The model under review builds one solid part; all positions refer to its coordinate system, in mm. A direction names the side the tool comes from. Round coordinates to 2 decimals unless told otherwise and drop trailing zeros. Order: outer loops, then holes, each group sorted by start corner. A loop starts at its lowest first (then second) coordinate and runs counter-clockwise, first axis right, second up. Notation, with made-up numbers: M 51,75 L 99,75 A18 ccw 99,106 Z; hole C 20.25,87 d11. An arc over 180 degrees is marked long. Use a Markdown table: item, result. Add a question column.
1. The part is to be moulded in two halves that separate along X. For faces 3 (the flat face through (-44.008, -8.908, 55.662)), 4 (the cylindrical face through (-14.31, -5.15, -55.94)), 5 (the flat face through (-44, -5, 56.914)), say which applies: +X half, -X half, draft (parallel to the pull), parting line (faces both ways), or undercut.
2. Insertion check: P1, Ø2, axis at y = -1.5, z = -33, coming from the -X side; P2, Ø2, axis at x = -40, z = -7, coming from the -Y side. Each pin has a flat end and moves straight along its axis. Give the tip position at first contact, or say it passes through.
3. For faces 1 (the flat face through (-45, -5, 54.374)), 2 (the cylindrical face through (-64.314, -1.252, 49.628)), list the 3-axis set-ups (+Z, -Z, +X, -X, +Y, -Y) from which the entire face can be reached by the end or side of a thin tool; tool diameter is ignored.
4. Consider section A-A on y = -6.5. State the section outline as (x, z) points.
5. To check wall thickness, follow probe 1 along Z at (x, y) = (-30, -3.25); probe 2 along X at (y, z) = (-3, 50); probe 3 along X at (y, z) = (-6.5, -52.5). State the ranges of each line that lie inside material, in increasing order.
6. Consider section B-B on x = -43. State the section outline as (y, z) points.
7. Consider section C-C on z = 15.5. State the section outline as (x, y) points.
from build123d import *

# Parameters (mm, degrees)
F1_DEPTH     = 12.7
F2_T         = -2.54
F3_R         = 5.08
F4_T1_DEPTH  = 109.2192415341
F4_T6_DEPTH  = 70.8878458195
F4_T11_DEPTH = 71.2857341695
F4_T16_DEPTH = 135.3482654479
F4_T23_DEPTH = 70.8878458195
F4_S24_R     = 5.08
F4_T25_DEPTH = 37
F4_T29_DEPTH = 135.3482654479
F4_S30_R     = 5.08
F4_T31_DEPTH = 69
F4_T38_DEPTH = 122.283391113
F4_S39_R     = 5.08
F4_T40_DEPTH = 63
F4_T44_DEPTH = 83.9519953984
F4_S45_R     = 5.08
F4_T46_DEPTH = 44
F4_T53_DEPTH = 84.3498837483
F4_S54_R     = 5.08
F4_T55_DEPTH = 44
F4_T59_DEPTH = 122.283391113
F4_S60_R     = 5.08
F4_T61_DEPTH = 63
F4_T68_DEPTH = 71.2857341695
F4_S69_R     = 5.08
F4_T70_DEPTH = 37
F4_T74_DEPTH = 135.3482654479
F4_S75_R     = 5.08
F4_T76_DEPTH = 69
F5_R         = 3.1205414485
F6_DEPTH     = 25.4


# Not quite as in the source:
# - a fillet or chamfer that OpenCascade refuses, or shapes differently, is made with other operations: its cross-section is extruded or revolved along the edge and cut away or added


with BuildPart() as f1:
    # F0 (on Front) → F1 (new body)
    with BuildSketch(Plane.XZ):
        Polygon((-76.0919898748, 56.9143295288), (-75.6755949615, -57.3849120053), (-12.7811351476, -57.3849120053), (-12.7811351476, 56.9143295288), align=None)
    extrude(amount=F1_DEPTH)

    # F2
    f2_openings = [f1.faces().sort_by_distance(p)[0] for p in [
        (-44.332578, -12.7, -0.172439),
    ]]
    offset(amount=F2_T, openings=f2_openings)

    # F3
    f3_edges = [f1.edges().sort_by_distance(p)[0] for p in [
        (-12.781135, -6.35, 56.91433),
        (-76.09199, -6.35, 56.91433),
        (-12.781135, -6.35, -57.384912),
        (-75.675595, -6.35, -57.384912),
    ]]
    fillet(f3_edges, radius=F3_R)

    # F4: chamfer of 5.08 on 4 edges, made by hand

    # F4_s2 → F4_t1 (cut)
    with BuildSketch(Plane.XY.offset(-54.8449120053)):
        Polygon((-10.2411351476, -12.7), (-15.3211351476, -7.62), (-15.3211351476, -12.7), align=None)
    extrude(amount=F4_T1_DEPTH, mode=Mode.SUBTRACT)


with BuildPart() as f4_tool4:
    # F4_s5 → F4_t6 (new body)
    with BuildSketch(Plane.YZ.offset(-86.2089809671)):
        Polygon((-12.7, -59.9249120053), (-7.62, -54.8449120053), (-12.7, -54.8449120053), align=None)
    extrude(amount=F4_T6_DEPTH)

    split(bisect_by=Plane(origin=(-73.3436593453, 0, -0.2671927326), x_dir=(0, 1, 0), z_dir=(0.9999933643, 0, 0.0036430001)), keep=Keep.TOP)


with BuildPart() as f1_1:
    add(f1.part)

    # F4_t3: cut F4_tool4
    add(f4_tool4.part, mode=Mode.SUBTRACT)


with BuildPart() as f4_tool9:
    # F4_s10 → F4_t11 (new body)
    with BuildSketch(Plane.YZ.offset(-15.3211351476)):
        Polygon((-12.7, 59.4543295288), (-7.62, 54.3743295288), (-12.7, 54.3743295288), align=None)
    extrude(amount=-F4_T11_DEPTH)

    split(bisect_by=Plane(origin=(-73.3436593453, 0, -0.2671927326), x_dir=(0, 1, 0), z_dir=(0.9999933643, 0, 0.0036430001)), keep=Keep.TOP)


with BuildPart() as f1_2:
    add(f1_1.part)

    # F4_t8: cut F4_tool9
    add(f4_tool9.part, mode=Mode.SUBTRACT)


with BuildPart() as f4_tool14:
    # F4_s15 → F4_t16 (new body)
    with BuildSketch(Plane(origin=(-0.2466530914, 0, 67.7055851499), x_dir=(0, 1, 0), z_dir=(0.0036430001, 0, -0.9999933643))):
        Polygon((-12.7, -78.4241460385), (-7.62, -73.3441460385), (-12.7, -73.3441460385), align=None)
    extrude(amount=F4_T16_DEPTH)

    split(bisect_by=Plane.XY.offset(54.3743295288), keep=Keep.BOTTOM)

    split(bisect_by=Plane.XY.offset(-54.8449120053), keep=Keep.TOP)


with BuildPart() as f1_3:
    add(f1_2.part)

    # F4_t13: cut F4_tool14
    add(f4_tool14.part, mode=Mode.SUBTRACT)


with BuildPart() as f4_tool21:
    # F4_s22 → F4_t23 (new body)
    with BuildSketch(Plane.YZ.offset(-86.2089809671)):
        Polygon((-12.7, -59.9249120053), (-7.62, -54.8449120053), (-12.7, -54.8449120053), align=None)
    extrude(amount=F4_T23_DEPTH)

    # F4_s24 → F4_t25 (intersect, symmetric)
    with BuildSketch(Plane.XZ.offset(10.2)):
        with Locations((-70.614067815, -52.3049120053)):
            Circle(F4_S24_R)
    extrude(amount=F4_T25_DEPTH, both=True, mode=Mode.INTERSECT)

    split(bisect_by=Plane(origin=(-73.3436593453, 0, -0.2671927326), x_dir=(0, 1, 0), z_dir=(-0.9999933643, 0, -0.0036430001)), keep=Keep.TOP)


with BuildPart() as f4_tool27:
    # F4_s28 → F4_t29 (new body)
    with BuildSketch(Plane(origin=(-0.2466530914, 0, 67.7055851499), x_dir=(0, 1, 0), z_dir=(0.0036430001, 0, -0.9999933643))):
        Polygon((-12.7, -78.4241460385), (-7.62, -73.3441460385), (-12.7, -73.3441460385), align=None)
    extrude(amount=F4_T29_DEPTH)

    # F4_s30 → F4_t31 (intersect, symmetric)
    with BuildSketch(Plane.XZ.offset(10.2)):
        with Locations((-70.614067815, -52.3049120053)):
            Circle(F4_S30_R)
    extrude(amount=F4_T31_DEPTH, both=True, mode=Mode.INTERSECT)

    split(bisect_by=Plane.XY.offset(-54.8449120053), keep=Keep.BOTTOM)


with BuildPart() as f4_tool21_1:
    add(f4_tool21.part)

    # F4_t33: intersect F4_tool27
    add(f4_tool27.part, mode=Mode.INTERSECT)


with BuildPart() as f1_4:
    add(f1_3.part)

    # F4_t19: cut F4_tool21
    add(f4_tool21_1.part, mode=Mode.SUBTRACT)


with BuildPart() as f4_tool36:
    # F4_s37 → F4_t38 (new body)
    with BuildSketch(Plane.XY.offset(-67.9090615842)):
        Polygon((-10.2411351476, -12.7), (-15.3211351476, -7.62), (-15.3211351476, -12.7), align=None)
    extrude(amount=F4_T38_DEPTH)

    # F4_s39 → F4_t40 (intersect, symmetric)
    with BuildSketch(Plane.XZ.offset(10.2)):
        with Locations((-17.8611351476, -52.3049120053)):
            Circle(F4_S39_R)
    extrude(amount=F4_T40_DEPTH, both=True, mode=Mode.INTERSECT)

    split(bisect_by=Plane.XY.offset(-54.8449120053), keep=Keep.BOTTOM)


with BuildPart() as f4_tool42:
    # F4_s43 → F4_t44 (new body)
    with BuildSketch(Plane.YZ.offset(-86.2089809671)):
        Polygon((-12.7, -59.9249120053), (-7.62, -54.8449120053), (-12.7, -54.8449120053), align=None)
    extrude(amount=F4_T44_DEPTH)

    # F4_s45 → F4_t46 (intersect, symmetric)
    with BuildSketch(Plane.XZ.offset(10.2)):
        with Locations((-17.8611351476, -52.3049120053)):
            Circle(F4_S45_R)
    extrude(amount=F4_T46_DEPTH, both=True, mode=Mode.INTERSECT)

    split(bisect_by=Plane.YZ.offset(-15.3211351476), keep=Keep.TOP)


with BuildPart() as f4_tool36_1:
    add(f4_tool36.part)

    # F4_t48: intersect F4_tool42
    add(f4_tool42.part, mode=Mode.INTERSECT)


with BuildPart() as f1_5:
    add(f1_4.part)

    # F4_t34: cut F4_tool36
    add(f4_tool36_1.part, mode=Mode.SUBTRACT)


with BuildPart() as f4_tool51:
    # F4_s52 → F4_t53 (new body)
    with BuildSketch(Plane.YZ.offset(-2.2569855688)):
        Polygon((-12.7, 59.4543295288), (-7.62, 54.3743295288), (-12.7, 54.3743295288), align=None)
    extrude(amount=-F4_T53_DEPTH)

    # F4_s54 → F4_t55 (intersect, symmetric)
    with BuildSketch(Plane.XZ.offset(10.2)):
        with Locations((-17.8611351476, 51.8343295288)):
            Circle(F4_S54_R)
    extrude(amount=F4_T55_DEPTH, both=True, mode=Mode.INTERSECT)

    split(bisect_by=Plane.YZ.offset(-15.3211351476), keep=Keep.TOP)


with BuildPart() as f4_tool57:
    # F4_s58 → F4_t59 (new body)
    with BuildSketch(Plane.XY.offset(-54.8449120053)):
        Polygon((-10.2411351476, -12.7), (-15.3211351476, -7.62), (-15.3211351476, -12.7), align=None)
    extrude(amount=F4_T59_DEPTH)

    # F4_s60 → F4_t61 (intersect, symmetric)
    with BuildSketch(Plane.XZ.offset(10.2)):
        with Locations((-17.8611351476, 51.8343295288)):
            Circle(F4_S60_R)
    extrude(amount=F4_T61_DEPTH, both=True, mode=Mode.INTERSECT)

    split(bisect_by=Plane.XY.offset(54.3743295288), keep=Keep.TOP)


with BuildPart() as f4_tool51_1:
    add(f4_tool51.part)

    # F4_t63: intersect F4_tool57
    add(f4_tool57.part, mode=Mode.INTERSECT)


with BuildPart() as f1_6:
    add(f1_5.part)

    # F4_t49: cut F4_tool51
    add(f4_tool51_1.part, mode=Mode.SUBTRACT)


with BuildPart() as f4_tool66:
    # F4_s67 → F4_t68 (new body)
    with BuildSketch(Plane.YZ.offset(-15.3211351476)):
        Polygon((-12.7, 59.4543295288), (-7.62, 54.3743295288), (-12.7, 54.3743295288), align=None)
    extrude(amount=-F4_T68_DEPTH)

    # F4_s69 → F4_t70 (intersect, symmetric)
    with BuildSketch(Plane.XZ.offset(10.2)):
        with Locations((-70.9934496016, 51.8343295288)):
            Circle(F4_S69_R)
    extrude(amount=F4_T70_DEPTH, both=True, mode=Mode.INTERSECT)

    split(bisect_by=Plane(origin=(-73.3436593453, 0, -0.2671927326), x_dir=(0, 1, 0), z_dir=(-0.9999933643, 0, -0.0036430001)), keep=Keep.TOP)


with BuildPart() as f4_tool72:
    # F4_s73 → F4_t74 (new body)
    with BuildSketch(Plane(origin=(-0.2466530914, 0, 67.7055851499), x_dir=(0, 1, 0), z_dir=(0.0036430001, 0, -0.9999933643))):
        Polygon((-12.7, -78.4241460385), (-7.62, -73.3441460385), (-12.7, -73.3441460385), align=None)
    extrude(amount=F4_T74_DEPTH)

    # F4_s75 → F4_t76 (intersect, symmetric)
    with BuildSketch(Plane.XZ.offset(10.2)):
        with Locations((-70.9934496016, 51.8343295288)):
            Circle(F4_S75_R)
    extrude(amount=F4_T76_DEPTH, both=True, mode=Mode.INTERSECT)

    split(bisect_by=Plane.XY.offset(54.3743295288), keep=Keep.TOP)


with BuildPart() as f4_tool66_1:
    add(f4_tool66.part)

    # F4_t78: intersect F4_tool72
    add(f4_tool72.part, mode=Mode.INTERSECT)


with BuildPart() as f1_7:
    add(f1_6.part)

    # F4_t64: cut F4_tool66
    add(f4_tool66_1.part, mode=Mode.SUBTRACT)

    # F5 (on face) → F6 (cut)
    with BuildSketch(Plane(origin=(0, 0, 0), x_dir=(-1, 0, 0), z_dir=(0, 1, 0))):
        with Locations((67.4311071634, 49.4907200336)):
            Circle(F5_R)
    extrude(amount=-F6_DEPTH, mode=Mode.SUBTRACT)


solid = f1_7.part
Answer block:
| question | item | result |
|---|---|---|
| 1 | face 3 | undercut |
| 1 | face 4 | +X half |
| 1 | face 5 | draft |
| 2 | P1 | x = -75.77 |
| 2 | P2 | y = -2.54 |
| 3 | face 1 | -Y |
| 3 | face 2 | +Y, -Y |
| 4 | outline | M -76.07,51.82 L -75.69,-52.32 A5.08 ccw -70.61,-57.38 L -17.86,-57.38 A5.08 ccw -12.78,-52.3 L -12.78,51.83 A5.08 ccw -17.86,56.91 L -70.99,56.91 A5.08 ccw Z; hole M -73.54,54.37 L -73.14,-54.84 L -15.32,-54.84 L -15.32,54.37 Z |
| 5 | probe 1 | -57.38 to -54.84, 54.37 to 56.91 |
| 5 | probe 2 | -76.07 to -73.53, -15.32 to -12.78 |
| 5 | probe 3 | -75.69 to -73.15, -15.32 to -12.78 |
| 6 | outline | M -10.16,-57.38 L 0,-57.38 L 0,56.91 L -10.16,56.91 L -7.62,54.37 L -2.54,54.37 L -2.54,-54.84 L -7.62,-54.84 Z |
| 7 | outline | M -75.94,-10.16 L -73.4,-7.62 L -73.4,-2.54 L -15.32,-2.54 L -15.32,-7.62 L -12.78,-10.16 L -12.78,0 L -75.94,0 Z |
